Build history of the part. All positions in model axes, mm. A direction names the side the tool comes from. Coordinates: 2 decimals unless noted, no trailing zeros. Loops run counter-clockwise (first coordinate to the right, second up) from the corner with the lowest first, then second, coordinate; pieces in that order, holes last.
(1) Slice it at C-C (z = 31). Give the cut face in (x, y) (1 decimal).
(2) Flat gauge pins, fed straight in: P1, Ø12, axis at x = 4.5, y = -4, coming from the -Z side; P2, Ø1.1, axis at y = 14, z = 70.5, coming from the -X side; P3, Ø0.7, axis at y = 14, z = 58, coming from the +X side; P4, Ø6, axis at y = 11.5, z = 26, coming from the -X side. Where does each tip first touch, or does it go through?
(3) Slice it at D-D (x = 6.5). Give the cut face in (y, z), and give its area (3 significant figures).
(4) Wall check: L1, parallel to X at y = 0, z = 68; L2, parallel to Y at x = 2.5, z = 59; L3, parallel to Y at x = 10, z = 55. Give the ranges that are in metal, low to high.
(5) Tool access for faces 1 (the face through (-1.1, 12.2, 0)), 2 (the face through (-9.693, 12, 50)): list every direction of +Z, -Z, +X, -X, +Y, -Y with a clear straight run to the whole face (end or side of a thin tool).
(6) Slice it at A-A (y = 5). Give the cut face in (x, z), and give its area (3 significant figures).
(7) Slice it at B-B (x = 2.25). Give the cut face in (y, z).
from build123d import *

# Parameters (mm, degrees)
F0_W     = 8.8289421401
F0_H     = 1.353359101
F0_W_2   = 8.8226038183
F1_DEPTH = 101.6
F3_DEPTH = 25.4


with BuildPart() as f1:
    # F0 (on Top) → F1 (new body)
    with BuildSketch(Plane.XY):
        with Locations((5.1440017123, 14.0243795505)):
            Rectangle(F0_W, F0_H)
        with Locations((-5.2819712669, 14.0243795505)):
            Rectangle(F0_W_2, F0_H)
        with BuildLine():
            Line((-9.693273176, 13.3477), (-9.693273176, 9.1761402793))
            ThreePointArc((-9.693273176, 9.1761402793), (-5.67367671, 12.0818246917), (-0.8706693577, 13.319272884))
            Line((-0.8706693577, 13.319272884), (-0.8706693577, 13.3477))
            Line((-0.8706693577, 13.3477), (-9.693273176, 13.3477))
        make_face()
        with BuildLine():
            Line((-9.693273176, 9.1761402793), (-9.693273176, 6.6365813025))
            ThreePointArc((-9.693273176, 6.6365813025), (-5.8606559871, 10.1811820361), (-0.8706693577, 11.7151906139))
            Line((-0.8706693577, 11.7151906139), (-0.8706693577, 13.319272884))
            ThreePointArc((-0.8706693577, 13.319272884), (-5.67367671, 12.0818246917), (-9.693273176, 9.1761402793))
        make_face()
        with BuildLine():
            ThreePointArc((0.7295306423, 13.3277485095), (5.5211714169, 12.152273922), (9.5584727824, 9.3164742987))
            Line((9.5584727824, 9.3164742987), (9.5584727824, 13.3477))
            Line((9.5584727824, 13.3477), (0.7295306423, 13.3477))
            Line((0.7295306423, 13.3477), (0.7295306423, 13.3277485095))
        make_face()
        with BuildLine():
            ThreePointArc((0.7295306423, 11.7248258534), (5.6966915069, 10.2738241237), (9.5584727824, 6.8293011589))
            Line((9.5584727824, 6.8293011589), (9.5584727824, 9.3164742987))
            ThreePointArc((9.5584727824, 9.3164742987), (5.5211714169, 12.152273922), (0.7295306423, 13.3277485095))
            Line((0.7295306423, 13.3277485095), (0.7295306423, 11.7248258534))
        make_face()
        with BuildLine():
            ThreePointArc((11.7475, 0), (-3.4736169632, -11.2221986011), (-9.693273176, 6.6365813025))
            Line((-9.693273176, 6.6365813025), (-9.693273176, 9.1761402793))
            ThreePointArc((-9.693273176, 9.1761402793), (-4.9385318121, -12.4004838144), (13.3477, 0))
            ThreePointArc((13.3477, 0), (12.3641563086, 5.0287905172), (9.5584727824, 9.3164742987))
            Line((9.5584727824, 9.3164742987), (9.5584727824, 6.8293011589))
            ThreePointArc((9.5584727824, 6.8293011589), (11.1868654068, 3.5857772685), (11.7475, 0))
        make_face()
    extrude(amount=F1_DEPTH)


with BuildPart() as f3:
    # F2 (on Front) → F3 (new body)
    with BuildSketch(Plane.XZ):
        with BuildLine():
            ThreePointArc((4.0005, 82.55), (-2.8287806781, 85.3787806781), (0, 78.5495))
            ThreePointArc((0, 78.5495), (2.8287806781, 79.7212193219), (4.0005, 82.55))
        make_face()
    extrude(amount=F3_DEPTH)


with BuildPart() as f3b:
    # F2 (on Front) → F3, piece 2 (new body)
    with BuildSketch(Plane.XZ):
        with BuildLine():
            ThreePointArc((0, 10.3505), (-2.8287806781, 3.5212193219), (4.0005, 6.35))
            ThreePointArc((4.0005, 6.35), (2.8287806781, 9.1787806781), (0, 10.3505))
        make_face()
    extrude(amount=F3_DEPTH)


with BuildPart() as f1_1:
    add(f1.part)

    # F4: cut F3, F3b
    add(f3.part, mode=Mode.SUBTRACT)
    add(f3b.part, mode=Mode.SUBTRACT)


solid = f1_1.part
Response values:
1. outline: (-9.7, 9.2) arc R13.3 ccw (long way) to (9.6, 9.3) - (9.6, 14.7) - (0.7, 14.7) - (0.7, 11.7) arc R11.7 cw (long way) to (-0.9, 11.7) - (-0.9, 14.7) - (-9.7, 14.7) - close
2. P1: stops at z = 0
2. P2: stops at x = -9.69
2. P3: stops at x = 9.56
2. P4: stops at x = -10.29
3. outline: (-11.66, 0) - (-9.79, 0) - (-9.79, 101.6) - (-11.66, 101.6) - close; (9.79, 0) - (14.7, 0) - (14.7, 101.6) - (9.79, 101.6) - close
3. area: 690 mm2
4. L1: x = -13.35 to -11.75, 11.75 to 13.35
4. L2: y = -13.11 to -11.48, 11.48 to 14.7
4. L3: y = -8.84 to -6.16, 6.16 to 8.84
5. face 1: -Z, +X, -X, +Y, -Y
5. face 2: +Z, -Z, -X, +Y
6. outline: (-12.38, 0) - (-10.63, 0) - (-10.63, 101.6) - (-12.38, 101.6) - close; (10.63, 0) - (12.38, 0) - (12.38, 101.6) - (10.63, 101.6) - close
6. area: 355 mm2
7. outline: (-13.16, 0) - (-11.53, 0) - (-11.53, 3.04) - (-13.16, 3.04) - close; (-13.16, 9.66) - (-11.53, 9.66) - (-11.53, 79.24) - (-13.16, 79.24) - close; (-13.16, 85.86) - (-11.53, 85.86) - (-11.53, 101.6) - (-13.16, 101.6) - close; (11.53, 0) - (14.7, 0) - (14.7, 101.6) - (11.53, 101.6) - close
